```python
from build123d import *

# Parameters (mm, degrees)
ESBO_O2_R                     = 6
RESSALTO_EXTRUS_O1_DEPTH      = 20
ESBO_O3_R                     = 11
RESSALTO_EXTRUS_O2_DEPTH      = 350
FILETE1_R                     = 10
FILETE2_R                     = 5
RESSALTO_EXTRUS_O3_DEPTH      = 20
RESSALTO_EXTRUS_O4_START      = -5
ESBO_O7_R                     = 12
RESSALTO_EXTRUS_O4_DEPTH      = 5
FILETE3_R                     = 5
RESSALTO_EXTRUS_O5_DEPTH      = 40
RESSALTO_EXTRUS_O5_DEPTH_BACK = 10
FILETE4_R                     = 10
ESBO_O11_W                    = 23
ESBO_O11_H                    = 42.858571571
CORTE_EXTRUS_O3_DEPTH         = 40
FILETE5_R                     = 10
FILETE6_R                     = 1.5


with BuildPart() as part:
    # Esboço1 → Revolução1 (revolve)
    with BuildSketch(Plane.XY):
        with BuildLine():
            Line((-10, 0), (10, 0))
            ThreePointArc((10, 0), (0, 10), (-10, 0))
        make_face()
    revolve(axis=Axis((-10, 0, 0), (1, 0, 0)))

    # Esboço2 → Ressalto-extrusão1 (add)
    with BuildSketch(Plane(origin=(0, 0, 0), x_dir=(1, 0, 0), z_dir=(0, 1, 0))):
        with Locations(Location((0, 0, 0), (0, 0, 90))):
            Circle(ESBO_O2_R)
    extrude(amount=RESSALTO_EXTRUS_O1_DEPTH)

    # Esboço3 → Ressalto-extrusão2 (add)
    with BuildSketch(Plane(origin=(0, 20, 0), x_dir=(1, 0, 0), z_dir=(0, 1, 0))):
        with Locations(Location((0, 0, 0), (0, 0, 270))):
            Circle(ESBO_O3_R)
    extrude(amount=RESSALTO_EXTRUS_O2_DEPTH)

    # Filete1
    # the kernel refuses this fillet: 10 mm, written as the material it adds along each edge
    with BuildSketch(Plane(origin=(0, 20, 0), x_dir=(0, 0, -1), z_dir=(1, 0, 0))) as filete1_piece_1:
        with BuildLine():
            CenterArc((16, -8.660254038), FILETE1_R, 120, 60)
            Line((6, -8.660254038), (5.8, -8.660254038))
            Line((5.8, -8.660254038), (5.8, 0))
            Line((5.8, 0), (6, 0.2))
            ThreePointArc((6, 0.2), (8.5, 0.2), (10.9, 0.173205081))
            Line((10.9, 0.173205081), (11, 0))
        make_face()
    revolve(axis=Axis((0, 20, 0), (0, 1, 0)))

    # Filete2
    filete2_edges = [part.edges().sort_by_distance(p)[0] for p in [
        (11, 20, 0),
    ]]
    fillet(filete2_edges, radius=FILETE2_R)

    # Esboço5 → Ressalto-extrusão3 (add)
    with BuildSketch(Plane(origin=(0, 370, 0), x_dir=(1, 0, 0), z_dir=(0, 1, 0))):
        with BuildLine():
            Line((-8, -8.94427191), (-8, 0))
            ThreePointArc((-8, 0), (0, 8), (8, 0))
            Line((8, 0), (8, -8.94427191))
            ThreePointArc((8, -8.94427191), (12, 0), (8, 8.94427191))
            ThreePointArc((8, 8.94427191), (0, 12), (-8, 8.94427191))
            ThreePointArc((-8, 8.94427191), (-12, 0), (-8, -8.94427191))
        make_face()
    extrude(amount=RESSALTO_EXTRUS_O3_DEPTH)

    # Esboço7 → Ressalto-extrusão4 (add)
    with BuildSketch(Plane(origin=(0, 370, 0), x_dir=(1, 0, 0), z_dir=(0, 1, 0)).offset(RESSALTO_EXTRUS_O4_START)):
        with Locations(Location((0, 0, 0), (0, 0, 311.810314896))):
            Circle(ESBO_O7_R)
    extrude(amount=RESSALTO_EXTRUS_O4_DEPTH)

    # Filete3
    # the kernel refuses this fillet: 5 mm, written as the material it adds along each edge
    with BuildSketch(Plane(origin=(0, 365, 0), x_dir=(0, 0, 1), z_dir=(1, 0, 0))) as filete3_piece_1:
        with BuildLine():
            CenterArc((16, 3), FILETE3_R, 180, 36.869897646)
            Line((12, 0), (11.92, -0.06))
            ThreePointArc((11.92, -0.06), (11.5, -0.1), (11, -0.1))
            Line((11, -0.1), (10.9, 0))
            Line((10.9, 0), (10.9, 3))
            Line((10.9, 3), (11, 3))
        make_face()
    revolve(axis=Axis((0, 365, 0), (0, -1, 0)))

    # Esboço8 → Corte-Revolução1 (revolve, cut)
    with BuildSketch(Plane.XY):
        with BuildLine():
            Line((0, 368.32023385), (0, 388.32023385))
            ThreePointArc((0, 388.32023385), (-10, 378.32023385), (0, 368.32023385))
        make_face()
    revolve(axis=Axis((0, 368.32023385, 0), (0, 1, 0)), mode=Mode.SUBTRACT)

    # Esboço10 → Ressalto-extrusão5 (add, two sides: drawn at the far end of the back side and taken through both)
    with BuildSketch(Plane(origin=(0, 390, 0), x_dir=(1, 0, 0), z_dir=(0, 1, 0)).offset(-RESSALTO_EXTRUS_O5_DEPTH_BACK)):
        with BuildLine():
            Line((-8, -8.94427191), (-8, -12.68857754))
            ThreePointArc((-8, -12.68857754), (0, 15), (8, -12.68857754))
            Line((8, -12.68857754), (8, -8.94427191))
            ThreePointArc((8, -8.94427191), (0, 12), (-8, -8.94427191))
        make_face()
    extrude(amount=RESSALTO_EXTRUS_O5_DEPTH + RESSALTO_EXTRUS_O5_DEPTH_BACK)

    # Filete4
    # the kernel refuses this fillet: 10 mm, written as the material it takes off along each edge
    with BuildSketch(Plane(origin=(0, 380, 0), x_dir=(-0.003141587485879309, 0, 0.9999950652018582), z_dir=(0.9999950652018582, 0, 0.003141587485879309))) as filete4_piece_1:
        with BuildLine():
            CenterArc((5, -7.141428429), FILETE4_R, 0, 45.572995999)
            Line((15, -7.141428429), (15, 0))
            Line((15, 0), (12, 0))
        make_face()
    revolve(axis=Axis((0, 380, 0), (0, -1, 0)), revolution_arc=359.64, mode=Mode.SUBTRACT)

    # Esboço11 → Corte-extrusão3 (cut)
    with BuildSketch(Plane.XY):
        with Locations((0, 408.570714215)):
            Rectangle(ESBO_O11_W, ESBO_O11_H)
    extrude(amount=CORTE_EXTRUS_O3_DEPTH, mode=Mode.SUBTRACT)

    # Filete5
    # the kernel refuses this fillet: 10 mm, written as the material it adds along each edge
    with BuildSketch(Plane(origin=(11.5, 387.141428429, -18.998355192), x_dir=(-1, 0, 0), z_dir=(0, 0, 1))) as filete5_piece_1_section:
        with BuildLine():
            CenterArc((10, -7.599342077), FILETE5_R, 130.541601874, 49.458398126)
            Line((0, -7.599342077), (0, 0))
            Line((0, 0), (3.5, 0))
        make_face()
    filete5_piece_1 = extrude(amount=47.627390526, mode=Mode.PRIVATE)
    filete5_piece_1 = filete5_piece_1 & Plane(origin=(0, 388.451461542, 0), x_dir=(-0.5333333333333332, 0, 0.8459051693633014), z_dir=(0, -1, 0)) * Cylinder(15, 126, mode=Mode.PRIVATE)
    filete5_piece_1 = split(filete5_piece_1, bisect_by=Plane(origin=(9.300320043, 390, 4.472135955), z_dir=(0, -1, 0)), keep=Keep.TOP, mode=Mode.PRIVATE)
    add(filete5_piece_1)
    with BuildSketch(Plane(origin=(11.5, 387.141428429, -18.998355192), x_dir=(-1, 0, 0), z_dir=(0, 0, 1))) as filete5_piece_2_section:
        with BuildLine():
            CenterArc((10, -7.599342077), FILETE5_R, 130.541601874, 49.458398126)
            Line((0, -7.599342077), (0, 0))
            Line((0, 0), (3.5, 0))
        make_face()
    filete5_piece_2 = extrude(amount=47.627390526, mode=Mode.PRIVATE)
    filete5_piece_2 = filete5_piece_2 & Plane(origin=(0, 392.291329927, 0), x_dir=(-0.5333333333333332, 0, 0.8459051693633014), z_dir=(0, -1, 0)) * Cylinder(15, 126, mode=Mode.PRIVATE)
    filete5_piece_2 = filete5_piece_2 - Plane(origin=(0, 392.291329927, 0), x_dir=(0.666666666666667, 0, 0.7453559924999297), z_dir=(0, -1, 0)) * Cylinder(12, 126, mode=Mode.PRIVATE)
    add(filete5_piece_2)
    with BuildSketch(Plane(origin=(-11.5, 387.141428429, -18.998355192), x_dir=(1, 0, 0), z_dir=(0, 0, 1))) as filete5_piece_3_section:
        with BuildLine():
            CenterArc((10, 7.599342077), FILETE5_R, 180, 49.458398126)
            Line((0, 7.599342077), (0, 0))
            Line((0, 0), (3.5, 0))
        make_face()
    filete5_piece_3 = extrude(amount=47.627390526, mode=Mode.PRIVATE)
    filete5_piece_3 = filete5_piece_3 & Plane(origin=(0, 388.451461532, 0), x_dir=(-0.5333333333333332, 0, 0.8459051693633014), z_dir=(0, -1, 0)) * Cylinder(15, 126, mode=Mode.PRIVATE)
    filete5_piece_3 = split(filete5_piece_3, bisect_by=Plane(origin=(-9.300320034, 390, 4.472135955), z_dir=(0, -1, 0)), keep=Keep.TOP, mode=Mode.PRIVATE)
    add(filete5_piece_3)
    with BuildSketch(Plane(origin=(-11.5, 387.141428429, -18.998355192), x_dir=(1, 0, 0), z_dir=(0, 0, 1))) as filete5_piece_4_section:
        with BuildLine():
            CenterArc((10, 7.599342077), FILETE5_R, 180, 49.458398126)
            Line((0, 7.599342077), (0, 0))
            Line((0, 0), (3.5, 0))
        make_face()
    filete5_piece_4 = extrude(amount=47.627390526, mode=Mode.PRIVATE)
    filete5_piece_4 = filete5_piece_4 & Plane(origin=(0, 392.291329925, 0), x_dir=(-0.5333333333333332, 0, 0.8459051693633014), z_dir=(0, -1, 0)) * Cylinder(15, 126, mode=Mode.PRIVATE)
    filete5_piece_4 = filete5_piece_4 - Plane(origin=(0, 392.291329925, 0), x_dir=(0.666666666666667, 0, 0.7453559924999297), z_dir=(0, -1, 0)) * Cylinder(12, 126, mode=Mode.PRIVATE)
    add(filete5_piece_4)

    # Filete6
    filete6_edges = [part.edges().sort_by_distance(p)[0] for p in [
        (9.284750533, 388.464015043, 0),
        (-9.284750533, 388.464015043, 0),
    ]]
    fillet(filete6_edges, radius=FILETE6_R)


solid = part.part
```
CAD build for the part. Positions are in the model's coordinates, mm. A direction names the side the tool comes from. Round coordinates to 2 decimals unless told otherwise and drop trailing zeros. Order: outer loops, then holes, each group sorted by start corner. A loop starts at its lowest first (then second) coordinate and runs counter-clockwise, first axis right, second up.
Q1. Slice it at A-A (y = 64). Write the cut outline in (x, z), and give its area (3 significant figures).
Q2. Two-plate mould, pull along Y, no slides. Class faces 6 (the cylindrical face through (10.11, 389.655, 7.016)), 7 (the cylindrical face through (-1.802, 9.646, -5.723)), 8 (the cylindrical face through (0, 371, -8)): pulls with the +Y half, pulls with the -Y half, needs draft (parallel to the pull), parting line crosses it, or undercut.
Q3. Which spindle directions (+Z, -Z, +X, -X, +Y, -Y) get a long thin tool onto all of the face, cutting with end or side? Do faces 1 (the cylindrical face through (-0.54, 408.27, -14.99)), 2 (the cylindrical face through (0, 387, -8)), 3 (the cylindrical face through (-10.74, 189.88, -2.38)), 4 (the flat face through (2, 430, -12)), 5 (the flat face through (0.8, 390, -8.3)). Say none if no direction does.
Q4. Wall check: L1, parallel to X at y = 406, z = 0; L2, parallel to Y at x = 9, z = -1.5; L3, parallel to Z at x = -9.5, y = 351.5. Give the ranges that are in metal, low to high.
Q5. Drop flat-ended pins along their axis: pin 1 (1.5 mm diameter, centred on y = 374, z = 6, fed in from +X); pin 2 (1 mm diameter, centred on x = 0, z = 6.5, fed in from -Y); pin 3 (3 mm diameter, centred on x = -4, z = -2, fed in from -Y); pin 4 (5 mm diameter, centred on x = -1.5, z = -11.5, fed in from +Y). Give the stop position or say it passes through.
Results below:
1. outline: circle Ø22 at (0, 0)
1. area: 380 mm2
2. face 6: pulls with the +Y half
2. face 7: undercut
2. face 8: needs draft
3. face 1: +Y, -Y
3. face 2: +Z, +Y
3. face 3: -Y
3. face 4: +Z, -Z, +X, -X, +Y
3. face 5: +Y
4. L1: x = -15 to -12, 12 to 15
4. L2: y = -4.09 to 4.09, 18.6 to 374.23, 382.41 to 390
4. L3: z = -5.55 to 5.55
5. pin 1: stops at x = 10.79
5. pin 2: stops at y = -8
5. pin 3: stops at y = -9.55
5. pin 4: stops at y = 430
